Build history of the part. All positions in model axes, mm. Face numbers are marked on the shaded views. A direction names the side the tool comes from. Coordinates: 2 decimals unless noted, no trailing zeros. Loops run counter-clockwise (first coordinate to the right, second up) from the corner with the lowest first, then second, coordinate; pieces in that order, holes last.
(1) Tool access for the marked faces 1, 2 and 3: list every direction of +Z, -Z, +X, -X, +Y, -Y with a clear straight run to the whole face (end or side of a thin tool).
(2) Slice it at D-D (z = 52.5). Give the cut face in (x, y), and give its area (3 significant figures).
(3) Two-plate mould, pull along X, no slides. Class the marked faces 4, 5 and 6: pulls with the +X half, pulls with the -X half, needs draft (parallel to the pull), parting line crosses it, or undercut.
(4) Slice it at A-A (y = 67.5). Give the cut face in (x, z).
(5) Flat gauge pins, fed straight in: P1, Ø1.5, axis at x = -2, z = -16, coming from the +Y side; P2, Ø23, axis at y = 52.5, z = 12.5, coming from the -X side; P3, Ø10, axis at x = -57.5, z = 32.5, coming from the -Y side. Where does each tip first touch, or does it go through?
(6) Slice it at C-C (x = -31). Give the cut face in (y, z), and give its area (3 significant figures).
(7) Slice it at B-B (z = -3.5). Give the cut face in (x, y), and give its area (3 significant figures).
(8) Wall check: L1, parallel to Z at x = -4, y = 76; L2, parallel to Z at x = -23.5, y = 79.5. Give the ranges that are in metal, low to high.
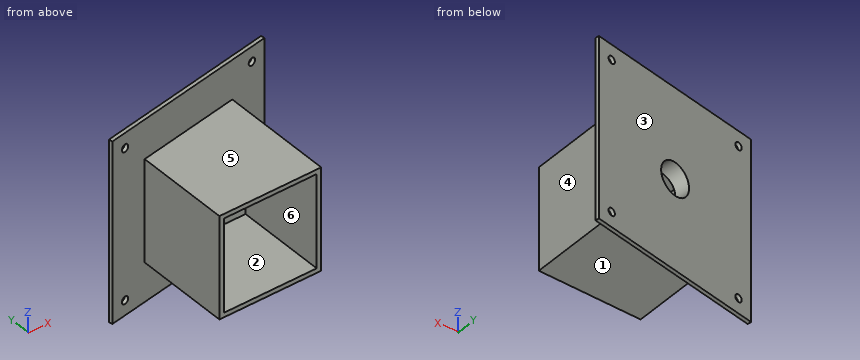
from build123d import *

# Parameters (mm, degrees)
SKETCH1_W                       = 86.36
SKETCH1_H                       = 86.36
BOSS_EXTRUDE1_DEPTH             = 95.25
SKETCH2_W                       = 78.74
SKETCH2_H                       = 78.74
CUT_EXTRUDE1_DEPTH              = 76.2
CUT_EXTRUDE2_DEPTH              = 87.36
SKETCH7_W                       = 152.4
SKETCH7_H                       = 152.4
BOSS_EXTRUDE2_DEPTH             = 3.175
SKETCH9_R                       = 13.97
CUT_EXTRUDE4_DEPTH              = 103.510777623
F_1_4_0_25_DIAMETER_HOLE1_D     = 6.35
F_1_4_0_25_DIAMETER_HOLE1_DEPTH = 3.175
F_1_4_0_25_DIAMETER_HOLE1_TIP   = 1.907732465


with BuildPart() as part:
    # Sketch1 → Boss-Extrude1 (new body)
    with BuildSketch(Plane(origin=(0, 0, 0), x_dir=(1, 0, 0), z_dir=(0, 1, 0))):
        Rectangle(SKETCH1_W, SKETCH1_H)
    extrude(amount=BOSS_EXTRUDE1_DEPTH)

    # Sketch2 → Cut-Extrude1 (cut)
    with BuildSketch(Plane(origin=(0, 0, 0), x_dir=(-1, 0, 0), z_dir=(0, -1, 0))):
        Rectangle(SKETCH2_W, SKETCH2_H)
    extrude(amount=-CUT_EXTRUDE1_DEPTH, mode=Mode.SUBTRACT)

    # Sketch4 → Cut-Extrude2 (cut, through all)
    with BuildSketch(Plane(origin=(0, 0, -43.18), x_dir=(-1, 0, 0), z_dir=(0, 0, -1))):
        Polygon((-43.18, 95.25), (43.18, 80.022401946), (43.18, 95.25), align=None)
    extrude(amount=-CUT_EXTRUDE2_DEPTH, mode=Mode.SUBTRACT)

    # Sketch7 → Boss-Extrude2 (add)
    with BuildSketch(Plane(origin=(-14.986673009, 84.993646171, 0), x_dir=(0.984807753, 0.173648178, 0), z_dir=(-0.173648178, 0.984807753, 0))):
        with Locations((15.217866597, 0)):
            Rectangle(SKETCH7_W, SKETCH7_H)
    extrude(amount=BOSS_EXTRUDE2_DEPTH)

    # Sketch9 → Cut-Extrude4 (cut, through all)
    with BuildSketch(Plane(origin=(-15.538005973, 88.120410786, 0), x_dir=(0.984807753, 0.173648178, 0), z_dir=(-0.173648178, 0.984807753, 0))):
        with Locations((15.217866597, 0)):
            Circle(SKETCH9_R)
    extrude(amount=-CUT_EXTRUDE4_DEPTH, mode=Mode.SUBTRACT)

    # 1/4 (0.25) Diameter Hole1
    with Locations(Plane(origin=(-15.538005973, 88.120410786, 0), x_dir=(0.984807753, 0.173648178, 0), z_dir=(-0.173648178, 0.984807753, 0))):
        with Locations((-48.282133403, 63.5), (78.717866597, 63.5), (78.717866597, -63.5), (-48.282133403, -63.5)):
            Hole(F_1_4_0_25_DIAMETER_HOLE1_D / 2, depth=F_1_4_0_25_DIAMETER_HOLE1_DEPTH)
            with Locations((0, 0, -(F_1_4_0_25_DIAMETER_HOLE1_DEPTH + F_1_4_0_25_DIAMETER_HOLE1_TIP / 2))):  # 118° drill point
                Cone(0, F_1_4_0_25_DIAMETER_HOLE1_D / 2, F_1_4_0_25_DIAMETER_HOLE1_TIP, mode=Mode.SUBTRACT)


solid = part.part
Response values:
1. face 1: -Z, +X, -Y
1. face 2: -Y
1. face 3: +Z, -Z, -X, +Y
2. outline: (-75.59, 77.53) - (-75.04, 74.4) - (75.04, 100.87) - (74.49, 103.99) - close
2. area: 484 mm2
3. face 4: pulls with the +X half
3. face 5: needs draft
3. face 6: undercut
4. outline: (-43.18, -43.18) - (43.18, -43.18) - (43.18, 43.18) - (-43.18, 43.18) - close; hole (-39.37, -39.37) - (39.37, -39.37) - (39.37, 39.37) - (-39.37, 39.37) - close
5. P1: stops at y = 90.64
5. P2: stops at x = -43.18
5. P3: stops at y = 76.62
6. outline: (0, -43.18) - (82.17, -43.18) - (82.17, -76.2) - (85.39, -76.2) - (85.39, 76.2) - (82.17, 76.2) - (82.17, 43.18) - (0, 43.18) - (0, 39.37) - (76.2, 39.37) - (76.2, -39.37) - (0, -39.37) - close
6. area: 1,590 mm2
7. outline: (-75.59, 77.53) - (-75.04, 74.4) - (-43.18, 80.02) - (-43.18, 0) - (-39.37, 0) - (-39.37, 76.2) - (-11.72, 76.2) - (-13.87, 88.41) - close; (12.77, 93.11) - (15.75, 76.2) - (39.37, 76.2) - (39.37, 0) - (43.18, 0) - (43.18, 95.25) - (75.04, 100.87) - (74.49, 103.99) - close
7. area: 1,650 mm2
8. L1: z = -43.18 to -39.37, 39.37 to 43.18
8. L2: z = -43.18 to 43.18
